from build123d import *

# Parameters (mm, degrees)
SKETCH_1_R      = 3.4
EXTRUDE_1_DEPTH = 1000


with BuildPart() as part:
    # Эскиз1 → Бобышка-Вытянуть1 (new body)
    with BuildSketch(Plane.XY):
        with BuildLine():
            Line((10.25, -20), (17.5, -20))
            ThreePointArc((17.5, -20), (19.267766953, -19.267766953), (20, -17.5))
            Line((20, -17.5), (20, -10.25))
            Line((20, -10.25), (20, -5.4))
            ThreePointArc((20, -5.4), (19.912132034, -5.187867966), (19.7, -5.1))
            Line((19.7, -5.1), (19.3, -5.1))
            ThreePointArc((19.3, -5.1), (19.087867966, -5.012132034), (19, -4.8))
            Line((19, -4.8), (19, -4.4))
            ThreePointArc((19, -4.4), (18.912132034, -4.187867966), (18.7, -4.1))
            Line((18.7, -4.1), (15.8, -4.1))
            ThreePointArc((15.8, -4.1), (15.587867966, -4.187867966), (15.5, -4.4))
            Line((15.5, -4.4), (15.5, -6.3))
            ThreePointArc((15.5, -6.3), (15.587867966, -6.512132034), (15.8, -6.6))
            Line((15.8, -6.6), (17, -6.6))
            ThreePointArc((17, -6.6), (17.707106781, -6.892893219), (18, -7.6))
            Line((18, -7.6), (18, -9.25))
            ThreePointArc((18, -9.25), (17.707106781, -9.957106781), (17, -10.25))
            Line((17, -10.25), (12.864213562, -10.25))
            ThreePointArc((12.864213562, -10.25), (12.48153013, -10.173879533), (12.157106781, -9.957106781))
            Line((12.157106781, -9.957106781), (7.992893219, -5.792893219))
            ThreePointArc((7.992893219, -5.792893219), (7.776120467, -5.46846987), (7.7, -5.085786438))
            Line((7.7, -5.085786438), (7.7, 5.085786438))
            ThreePointArc((7.7, 5.085786438), (7.776120467, 5.46846987), (7.992893219, 5.792893219))
            Line((7.992893219, 5.792893219), (12.157106781, 9.957106781))
            ThreePointArc((12.157106781, 9.957106781), (12.48153013, 10.173879533), (12.864213562, 10.25))
            Line((12.864213562, 10.25), (17, 10.25))
            ThreePointArc((17, 10.25), (17.707106781, 9.957106781), (18, 9.25))
            Line((18, 9.25), (18, 7.6))
            ThreePointArc((18, 7.6), (17.707106781, 6.892893219), (17, 6.6))
            Line((17, 6.6), (15.8, 6.6))
            ThreePointArc((15.8, 6.6), (15.587867966, 6.512132034), (15.5, 6.3))
            Line((15.5, 6.3), (15.5, 4.4))
            ThreePointArc((15.5, 4.4), (15.587867966, 4.187867966), (15.8, 4.1))
            Line((15.8, 4.1), (18.7, 4.1))
            ThreePointArc((18.7, 4.1), (18.912132034, 4.187867966), (19, 4.4))
            Line((19, 4.4), (19, 4.8))
            ThreePointArc((19, 4.8), (19.087867966, 5.012132034), (19.3, 5.1))
            Line((19.3, 5.1), (19.7, 5.1))
            ThreePointArc((19.7, 5.1), (19.912132034, 5.187867966), (20, 5.4))
            Line((20, 5.4), (20, 10.25))
            Line((20, 10.25), (20, 17.416573868))
            ThreePointArc((20, 17.416573868), (19.207825128, 19.242315726), (17.333333333, 19.911012126))
            ThreePointArc((17.333333333, 19.911012126), (-8.284271247, 8.284271247), (-19.911012126, -17.333333333))
            ThreePointArc((-19.911012126, -17.333333333), (-19.242315726, -19.207825128), (-17.416573868, -20))
            Line((-17.416573868, -20), (-10.25, -20))
            Line((-10.25, -20), (-5.4, -20))
            ThreePointArc((-5.4, -20), (-5.187867966, -19.912132034), (-5.1, -19.7))
            Line((-5.1, -19.7), (-5.1, -19.3))
            ThreePointArc((-5.1, -19.3), (-5.012132034, -19.087867966), (-4.8, -19))
            Line((-4.8, -19), (-4.4, -19))
            ThreePointArc((-4.4, -19), (-4.187867966, -18.912132034), (-4.1, -18.7))
            Line((-4.1, -18.7), (-4.1, -15.8))
            ThreePointArc((-4.1, -15.8), (-4.187867966, -15.587867966), (-4.4, -15.5))
            Line((-4.4, -15.5), (-6.3, -15.5))
            ThreePointArc((-6.3, -15.5), (-6.512132034, -15.587867966), (-6.6, -15.8))
            Line((-6.6, -15.8), (-6.6, -17))
            ThreePointArc((-6.6, -17), (-6.892893219, -17.707106781), (-7.6, -18))
            Line((-7.6, -18), (-9.25, -18))
            ThreePointArc((-9.25, -18), (-9.957106781, -17.707106781), (-10.25, -17))
            Line((-10.25, -17), (-10.25, -12.864213562))
            ThreePointArc((-10.25, -12.864213562), (-10.173879533, -12.48153013), (-9.957106781, -12.157106781))
            Line((-9.957106781, -12.157106781), (-5.792893219, -7.992893219))
            ThreePointArc((-5.792893219, -7.992893219), (-5.46846987, -7.776120467), (-5.085786438, -7.7))
            Line((-5.085786438, -7.7), (5.085786438, -7.7))
            ThreePointArc((5.085786438, -7.7), (5.46846987, -7.776120467), (5.792893219, -7.992893219))
            Line((5.792893219, -7.992893219), (9.957106781, -12.157106781))
            ThreePointArc((9.957106781, -12.157106781), (10.173879533, -12.48153013), (10.25, -12.864213562))
            Line((10.25, -12.864213562), (10.25, -17))
            ThreePointArc((10.25, -17), (9.957106781, -17.707106781), (9.25, -18))
            Line((9.25, -18), (7.6, -18))
            ThreePointArc((7.6, -18), (6.892893219, -17.707106781), (6.6, -17))
            Line((6.6, -17), (6.6, -15.8))
            ThreePointArc((6.6, -15.8), (6.512132034, -15.587867966), (6.3, -15.5))
            Line((6.3, -15.5), (4.4, -15.5))
            ThreePointArc((4.4, -15.5), (4.187867966, -15.587867966), (4.1, -15.8))
            Line((4.1, -15.8), (4.1, -18.7))
            ThreePointArc((4.1, -18.7), (4.187867966, -18.912132034), (4.4, -19))
            Line((4.4, -19), (4.8, -19))
            ThreePointArc((4.8, -19), (5.012132034, -19.087867966), (5.1, -19.3))
            Line((5.1, -19.3), (5.1, -19.7))
            ThreePointArc((5.1, -19.7), (5.187867966, -19.912132034), (5.4, -20))
            Line((5.4, -20), (10.25, -20))
        make_face()
        Circle(SKETCH_1_R, mode=Mode.SUBTRACT)
        with BuildLine():
            Line((18, 16.878177829), (18, 13.447331922))
            ThreePointArc((18, 13.447331922), (17.707106781, 12.740225141), (17, 12.447331922))
            Line((17, 12.447331922), (11.274711974, 12.447331922))
            ThreePointArc((11.274711974, 12.447331922), (-3.758787848, 3.758787848), (-12.447331922, -11.274711974))
            Line((-12.447331922, -11.274711974), (-12.447331922, -17))
            ThreePointArc((-12.447331922, -17), (-12.740225141, -17.707106781), (-13.447331922, -18))
            Line((-13.447331922, -18), (-16.878177829, -18))
            ThreePointArc((-16.878177829, -18), (-17.613392451, -17.677834389), (-17.874885338, -16.918918919))
            ThreePointArc((-17.874885338, -16.918918919), (-6.870057685, 6.870057685), (16.918918919, 17.874885338))
            ThreePointArc((16.918918919, 17.874885338), (17.677834389, 17.613392451), (18, 16.878177829))
        make_face(mode=Mode.SUBTRACT)
        with BuildLine():
            Line((13.2, -12.2), (17, -12.2))
            ThreePointArc((17, -12.2), (17.707106781, -12.492893219), (18, -13.2))
            Line((18, -13.2), (18, -17))
            ThreePointArc((18, -17), (17.707106781, -17.707106781), (17, -18))
            Line((17, -18), (13.2, -18))
            ThreePointArc((13.2, -18), (12.492893219, -17.707106781), (12.2, -17))
            Line((12.2, -17), (12.2, -13.2))
            ThreePointArc((12.2, -13.2), (12.492893219, -12.492893219), (13.2, -12.2))
        make_face(mode=Mode.SUBTRACT)
    extrude(amount=EXTRUDE_1_DEPTH)


solid = part.part
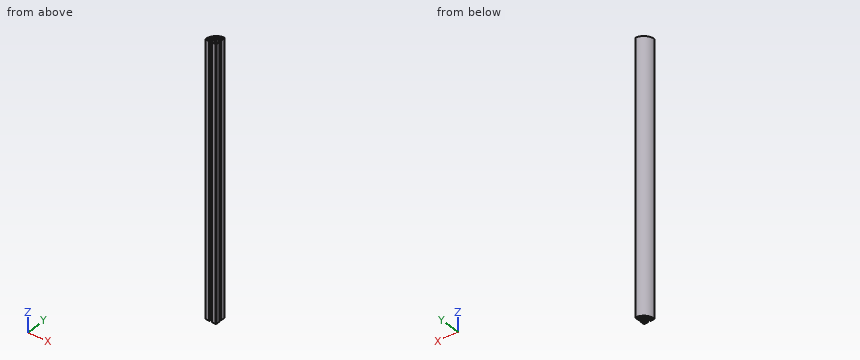
Input: part model. Units: mm. Frame: model coordinates. Give positions to 0.01 mm unless a question says otherwise; leave off trailing zeros.
Q1. Material intervals for probe 1 along Y at (x, z) = (11.5, 442.5); probe 2 along X at (y, z) = (-7.5, 934.5); probe 3 along X at (y, z) = (-8.5, 585.5), sorted ascending.
Q2. Section A-A, the plane z = 123. State how many separate pieces and enclosed holes the cut face has, plus the area to 3 significant figures.
Q3. First-contact query: P1, Ø1.3, axis at y = -8, z = 268, coming from the -X side; P2, Ø1.3, axis at y = 9, z = 459, coming from the -X side; P3, Ø10, axis at x = 6, z = 324, coming from the +Y side; P4, Ø1.5, axis at x = -9.5, y = 7.5, coming from the -Z side. Flat tips, straight axial feed; report the tip coordinate or a pass-through.
Filled in:
1. probe 1: y = -20 to -9.3, 9.3 to 12.45, 17.04 to 19.09
1. probe 2: x = -18 to -15.89, -11.19 to 9.7, 17.99 to 20
1. probe 3: x = -18.31 to -16.22, -11.57 to -6.3, 6.3 to 10.7, 18 to 20
2. separate pieces: 1
2. enclosed holes: 3
2. area: 558 mm2
3. P1: stops at x = -18.36
3. P2: stops at x = -8.22
3. P3: stops at y = 18.97
3. P4: stops at z = 0
